Design review of the part built by this model. Coordinates are the model's own, in mm. Face numbers are marked on the shaded views. A direction names the side the tool comes from. Coordinates: 2 decimals unless noted, no trailing zeros. Loops run counter-clockwise (first coordinate to the right, second up) from the corner with the lowest first, then second, coordinate; pieces in that order, holes last. Notation, with made-up numbers: M 83.5,-21.75 L 106.5,-21.75 A27 cw 106.5,8.25 Z; hole C 20.25,80.25 d11. An arc over 180 degrees is marked long. Write item = value, one per line. Start each with the question number.
```python
from build123d import *

# Parameters (mm, degrees)
F0_R     = 2
F0_R_2   = 1.75
F1_DEPTH = 5
F2_DEPTH = 7
F3_DEPTH = 3.2
F5_DEPTH = 3


with BuildPart() as f1:
    # F0 (on Top) → F1 (new body)
    with BuildSketch(Plane.XY):
        Polygon((0, -10.5), (19.29977, -10.5), (18.723261, 18.95), (0, 18.95), (-18.723261, 18.95), (-19.29977, -10.5), align=None)
        Polygon((-14.47088, -3.462027), (-16.483643, -0.024181), (-14.512763, 3.437846), (-10.52912, 3.462027), (-8.516357, 0.024181), (-10.487237, -3.437846), align=None, mode=Mode.SUBTRACT)
        Polygon((14.512763, 3.437846), (16.483643, -0.024181), (14.47088, -3.462027), (10.487237, -3.437846), (8.516357, 0.024181), (10.52912, 3.462027), align=None, mode=Mode.SUBTRACT)
        with Locations((-7.42, 6.15)):
            Circle(F0_R_2, mode=Mode.SUBTRACT)
        with Locations((7.42, 6.15)):
            Circle(F0_R_2, mode=Mode.SUBTRACT)
        Polygon((-14.512763, 3.437846), (-16.483643, -0.024181), (-14.47088, -3.462027), (-10.487237, -3.437846), (-8.516357, 0.024181), (-10.52912, 3.462027), align=None)
        with Locations((-12.5, 0)):
            Circle(F0_R, mode=Mode.SUBTRACT)
        Polygon((14.47088, -3.462027), (16.483643, -0.024181), (14.512763, 3.437846), (10.52912, 3.462027), (8.516357, 0.024181), (10.487237, -3.437846), align=None)
        with Locations((12.5, 0)):
            Circle(F0_R, mode=Mode.SUBTRACT)
    extrude(amount=F1_DEPTH)

    # F0 (on Top) → F2 (join)
    with BuildSketch(Plane.XY):
        Polygon((19.9, 20.15), (0, 20.15), (-19.9, 20.15), (-20.5, -10.5), (-19.29977, -10.5), (-18.723261, 18.95), (0, 18.95), (18.723261, 18.95), (19.29977, -10.5), (20.5, -10.5), align=None)
    extrude(amount=F2_DEPTH)

    # F0 (on Top) → F3 (cut)
    with BuildSketch(Plane.XY):
        Polygon((14.47088, -3.462027), (16.483643, -0.024181), (14.512763, 3.437846), (10.52912, 3.462027), (8.516357, 0.024181), (10.487237, -3.437846), align=None)
        with Locations((12.5, 0)):
            Circle(F0_R, mode=Mode.SUBTRACT)
        Polygon((-14.512763, 3.437846), (-16.483643, -0.024181), (-14.47088, -3.462027), (-10.487237, -3.437846), (-8.516357, 0.024181), (-10.52912, 3.462027), align=None)
        with Locations((-12.5, 0)):
            Circle(F0_R, mode=Mode.SUBTRACT)
    extrude(amount=F3_DEPTH, mode=Mode.SUBTRACT)

    # F4 (on face) → F5 (cut)
    with BuildSketch(Plane.XY.offset(5)):
        Polygon((10.653188, 6.14902), (9.03747, 8.949517), (5.804308, 8.950513), (4.186865, 6.15101), (5.802584, 3.350513), (9.035746, 3.349518), align=None)
        Polygon((-4.186865, 6.15101), (-5.804308, 8.950513), (-9.03747, 8.949517), (-10.653188, 6.14902), (-9.035746, 3.349518), (-5.802584, 3.350513), align=None)
    extrude(amount=-F5_DEPTH, mode=Mode.SUBTRACT)


solid = f1.part
```
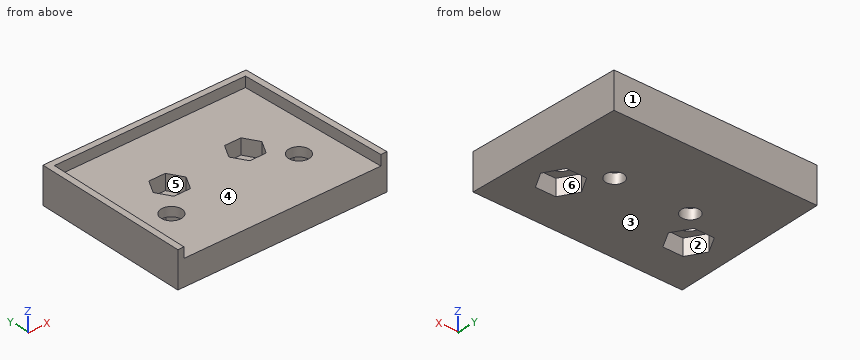
(1) Mouldability with a two-part tool opening along Y and no side actions: class the marked faces 1, 2 and 3 as +Y half, -Y half, draft (parallel to the pull), parting line (faces both ways), or undercut.
(2) Take a section at A-A (z = 1.25). State the section outline as (x, y) points.
(3) Take a section at D-D (x = -12.5). State the section outline as (y, z) points, plus the area to 3 significant figures.
(4) To check wall thickness, follow L1, parallel to X at y = 6.5, z = 1.5; L2, parallel to Y at x = 12.5, z = 3.6; L3, parallel to X at y = 1.5, z = 2. State the ranges of each line that lie inside material, in increasing order.
(5) Take a section at C-C (x = 8). State the section outline as (y, z) points, plus the area to 3 significant figures.
(6) Take a section at B-B (x = 0). State the section outline as (y, z) points.
(7) Insertion check: pin 1 (9 mm diameter, centred on x = 4, y = 2, fed in from +Z); pin 2 (4.5 mm diameter, centred on x = -7.42, y = 6.15, fed in from +Z); pin 3 (1.6 mm diameter, centred on x = 8, z = 6.5, fed in from -Y). Each pin has a flat end and moves straight along its axis. Give the tip position at first contact, or say it passes through.
(8) Tool access review of the marked faces 4, 5 and 6: name each direction out of +Z, -Z, +X, -X, +Y, -Y from which nothing blocks a thin tool from reaching the whole face with its end or side.
Results list:
q1.face_1 = +Y half
q1.face_2 = undercut
q1.face_3 = draft
q2.outline = M -20.5,-10.5 L 20.5,-10.5 L 19.9,20.15 L -19.9,20.15 Z; hole M -16.48,-0.02 L -14.47,-3.46 L -10.49,-3.44 L -8.52,0.02 L -10.53,3.46 L -14.51,3.44 Z; hole C -7.42,6.15 d3.5; hole C 7.42,6.15 d3.5; hole M 8.52,0.02 L 10.49,-3.44 L 14.47,-3.46 L 16.48,-0.02 L 14.51,3.44 L 10.53,3.46 Z
q3.outline = M -10.5,0 L -3.45,0 L -3.45,3.2 L -2,3.2 L -2,5 L -10.5,5 Z; M 2,3.2 L 3.45,3.2 L 3.45,0 L 20.15,0 L 20.15,7 L 18.95,7 L 18.95,5 L 2,5 Z
q3.area = 126 mm^2
q4.L1 = -20.17 to -9.13, -5.71 to 5.71, 9.13 to 20.17
q4.L2 = -10.5 to -2, 2 to 20.15
q4.L3 = -20.27 to -15.62, -9.38 to 9.38, 15.62 to 20.27
q5.outline = M -10.5,0 L 4.5,0 L 4.5,2 L 3.35,2 L 3.35,5 L -10.5,5 Z; M 7.8,0 L 20.15,0 L 20.15,7 L 18.95,7 L 18.95,5 L 8.95,5 L 8.95,2 L 7.8,2 Z
q5.area = 132 mm^2
q6.outline = M -10.5,0 L 20.15,0 L 20.15,7 L 18.95,7 L 18.95,5 L -10.5,5 Z
q7.pin_1 = 5
q7.pin_2 = 2
q7.pin_3 = 18.95
q8.face_4 = +Z, -Y
q8.face_5 = +Z
q8.face_6 = -Z
